Input: part model. Units: mm. Frame: model coordinates. Face numbers are marked on the shaded views. A direction names the side the tool comes from. Coordinates: 2 decimals unless noted, no trailing zeros. Order: outer loops, then holes, each group sorted by start corner. A loop starts at its lowest first (then second) coordinate and runs counter-clockwise, first axis right, second up. Notation, with made-up numbers: (49.5, -8.75) - (97.5, -8.75) arc R24 cw to (97.5, 30.25) - close; hole circle Ø11 at (7, 4.25). An arc over 180 degrees is marked (long way). Answer as CSV lines item,"result". Start each with the question number.
Item 1: Section B-B (y = 10). Output: boundary loops of the cut face in (x, z).
Item 2: Section A-A (z = 45). Output: boundary loops of the cut face in (x, y).
Item 3: First-contact query: pin 1 (6 mm diameter, centred on x = -7, y = 13, fed in from -Z). Flat tip, straight axial feed; report the tip coordinate or a pass-through.
Item 4: Material intervals for line 1 along Y through (x, z) = (-65, 41); line 2 along Z through (x, y) = (-40, 15.5); line 3 along X through (y, z) = (10.25, 46.5), sorted ascending.
Item 5: Section D-D (y = 2.5). Output: boundary loops of the cut face in (x, z).
Item 6: Section C-C (x = -40). Output: boundary loops of the cut face in (y, z).
Item 7: Access query for the marked faces 1, 2 and 3. Directions: +Z, -Z, +X, -X, +Y, -Y. A direction counts if a zero-diameter tool reaches every point of the face in a straight line with its end or side. Return the directions, or none.
Item 8: Draft query along Y for the marked faces 4, 5 and 6. Return one class per face: +Y half, -Y half, draft (parallel to the pull), parting line (faces both ways), or undercut.
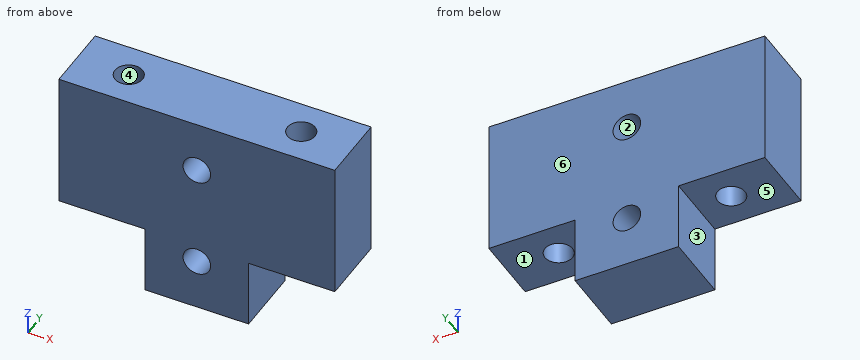
Autodesk Inventor part; units mm, degrees
ref_plane "YZ Plane" through (0, 0, 0) normal (1, 0, 0) x (0, 1, 0)
ref_plane "XZ Plane" through (0, 0, 0) normal (0, 1, 0) x (-1, 0, 0)
ref_plane "XY Plane" through (0, 0, 0) normal (0, 0, 1) x (1, 0, 0)
sketch "Sketch1" plane through (0, 0, 0) normal (0, 1, 0) x (-1, 0, 0)
  line L0 (0, 0) -> (80, 0)
  line L1 (80, 0) -> (80, 60)
  line L2 (80, 60) -> (0, 60)
  line L3 (0, 60) -> (0, 0)
  circle A0 centre (40, 45) radius 4
  circle A1 centre (40, 15) radius 4
  dimension "d0" = 80
  dimension "d1" = 60
  dimension "d4" = 8
  dimension "d5" = 8
extrude "Extrusion1" add sketch "Sketch1" along normal blind 20
sketch "Sketch2" plane through (-80, 0, 60) normal (0, 0, 1) x (1, 0, 0)
  circle A0 centre (15, 10) radius 4
  circle A1 centre (65, 10) radius 4
  dimension "d10" = 8
  dimension "d11" = 8
extrude "Extrusion2" cut sketch "Sketch2" against normal blind 60
sketch "Sketch3" plane through (0, 20, 0) normal (0, 1, 0) x (1, 0, 0)
  line L0 (0, 0) -> (-80, 0)
  line L1 (-80, 0) -> (-80, -60)
  line L2 (0, -60) -> (0, 0)
  line L3 (-40, 0) -> (-25, 0)
  line L4 (-40, 0) -> (-55, 0)
  line L5 (-80, -60) -> (-80, -20)
  line L6 (-80, -20) -> (-55, -20)
  line L7 (-55, -20) -> (-55, 0)
  line L8 (0, -20) -> (-25, -20)
  line L9 (-25, -20) -> (-25, 0)
  dimension "d14" = 15
  dimension "d15" = 15
  dimension "d16" = 40
extrude "Extrusion3" cut sketch "Sketch3" against normal blind 60
properties part number "X_Bottem_MotorSide_V3" material "Birch"
Determined:
1,outline,"(-80, 20) - (-69, 20) - (-69, 60) - (-80, 60) - close; (-61, 20) - (-55, 20) - (-55, 0) - (-25, 0) - (-25, 20) - (-19, 20) - (-19, 60) - (-61, 60) - close; (-11, 20) - (0, 20) - (0, 60) - (-11, 60) - close; hole circle Ø8 at (-40, 15); hole circle Ø8 at (-40, 45)"
2,outline,"(-80, 0) - (-44, 0) - (-44, 20) - (-80, 20) - close; (-36, 0) - (0, 0) - (0, 20) - (-36, 20) - close; hole circle Ø8 at (-65, 10); hole circle Ø8 at (-15, 10)"
3,pin 1,"stops at z = 20"
4,line 1,"y = 0 to 6, 14 to 20"
4,line 2,"z = 0 to 11, 19 to 41, 49 to 60"
4,line 3,"x = -80 to -68.99, -61.01 to -43.71, -36.29 to -18.99, -11.01 to 0"
5,outline,"(-80, 20) - (-55, 20) - (-55, 0) - (-25, 0) - (-25, 20) - (0, 20) - (0, 60) - (-80, 60) - close; hole circle Ø8 at (-40, 15); hole circle Ø8 at (-40, 45)"
6,outline,"(0, 0) - (20, 0) - (20, 11) - (0, 11) - close; (0, 19) - (20, 19) - (20, 41) - (0, 41) - close; (0, 49) - (20, 49) - (20, 60) - (0, 60) - close"
7,face 1,"-Z, +X, +Y, -Y"
7,face 2,"+Y, -Y"
7,face 3,"-Z, -X, +Y, -Y"
8,face 4,"undercut"
8,face 5,"draft"
8,face 6,"+Y half"
